```python
from build123d import *

# Parameters (mm, degrees)
MEMBER_1_DEPTH               = 1500
HOLE_WIZARD_M10_1_AT_2_COUNT = 2
HOLE_WIZARD_M10_1_AT_2_PITCH = 80
HOLE_WIZARD_M8_2_D           = 6.8
HOLE_WIZARD_M8_2_DEPTH       = 22.25
HOLE_WIZARD_M8_2_TIP         = 2.042926105


with BuildPart() as part:
    # Sketch11 → Member 1 (new body)
    with BuildSketch(Plane.YZ):
        with BuildLine():
            Line((-34, -40), (34, -40))
            ThreePointArc((34, -40), (38.242640687, -38.242640687), (40, -34))
            Line((40, -34), (40, 34))
            ThreePointArc((40, 34), (38.242640687, 38.242640687), (34, 40))
            Line((34, 40), (-34, 40))
            ThreePointArc((-34, 40), (-38.242640687, 38.242640687), (-40, 34))
            Line((-40, 34), (-40, -34))
            ThreePointArc((-40, -34), (-38.242640687, -38.242640687), (-34, -40))
        make_face()
        with BuildLine():
            Line((-34, -36), (34, -36))
            ThreePointArc((34, -36), (35.414213562, -35.414213562), (36, -34))
            Line((36, -34), (36, 34))
            ThreePointArc((36, 34), (35.414213562, 35.414213562), (34, 36))
            Line((34, 36), (-34, 36))
            ThreePointArc((-34, 36), (-35.414213562, 35.414213562), (-36, 34))
            Line((-36, 34), (-36, -34))
            ThreePointArc((-36, -34), (-35.414213562, -35.414213562), (-34, -36))
        make_face(mode=Mode.SUBTRACT)
    extrude(amount=MEMBER_1_DEPTH)

    # 草图4 → M10 间隙孔1 (revolve, cut)
    with BuildSketch(Plane(origin=(1380, 0, -36), x_dir=(0, -1, 0), z_dir=(1, 0, 0))):
        Polygon((0, 0), (0, 33.605163714), (6, 30), (6, 0), align=None)
    hole_wizard_m10_1 = revolve(axis=Axis((1380, 0, -29.65), (0, 0, -1)), mode=Mode.SUBTRACT)

    # M10 间隙孔1 at 2: M10 间隙孔1 ×2
    with Locations(*[(i * HOLE_WIZARD_M10_1_AT_2_PITCH, 0, 0) for i in range(1, HOLE_WIZARD_M10_1_AT_2_COUNT)]):
        add(hole_wizard_m10_1, mode=Mode.SUBTRACT)

    # 镜向1: M10 间隙孔1 across plane
    add(hole_wizard_m10_1.mirror(Plane.ZY.offset(-750)), mode=Mode.SUBTRACT)

    # 镜向1 copy 1 sketch → 镜向1 copy 1 (revolve, cut)
    with BuildSketch(Plane(origin=(40, 0, -36), x_dir=(0, -1, 0), z_dir=(-1, 0, 0))):
        Polygon((0, 0), (0, -33.605163714), (6, -30), (6, 0), align=None)
    revolve(axis=Axis((40, 0, -29.65), (0, 0, 1)), mode=Mode.SUBTRACT)

    # M8 螺纹孔2
    with Locations(Plane(origin=(0, 40, 0), x_dir=(-1, 0, 0), z_dir=(0, 1, 0))):
        with Locations((-100.000000009, 20), (-740.000000009, 20), (-1380.000000009, 20), (-1580.000000007, 20), (-2220.000000007, 20), (-2860.000000007, 20)):
            Hole(HOLE_WIZARD_M8_2_D / 2, depth=HOLE_WIZARD_M8_2_DEPTH)
            with Locations((0, 0, -(HOLE_WIZARD_M8_2_DEPTH + HOLE_WIZARD_M8_2_TIP / 2))):  # 118° drill point
                Cone(0, HOLE_WIZARD_M8_2_D / 2, HOLE_WIZARD_M8_2_TIP, mode=Mode.SUBTRACT)


solid = part.part
```
Geometry: final body of the model. Coordinates: model frame, mm. A direction names the side the tool comes from. Round coordinates to 2 decimals unless told otherwise and drop trailing zeros. Order: outer loops, then holes, each group sorted by start corner. A loop starts at its lowest first (then second) coordinate and runs counter-clockwise, first axis right, second up. Notation, with made-up numbers: (-17, -28.75) -> (12, -28.75) arc R15 cw to (12, -6.75) -> close; hole circle Ø9 at (24, -24). An arc over 180 degrees is marked (long way). Use CSV: the item, a comma, the result in double quotes. Start each with the question number.
1) Material intervals for line 1 along X through (y, z) = (0, -37.35); line 2 along Y through (x, z) = (414, -8.5), sorted ascending. Write a range as from..to.
2) Section B-B (x = 1339.5). Return the cut outline in (y, z), and give its area (3 significant figures).
3) Draft query along Z for faces 1 (the face through (740, 40, 0)), 2 (the face through (740, 0, -40)), 3 (the face through (740, 0, 36)). Return one class per face: +Z half, -Z half, draft (parallel to the pull), parting line (faces both ways), or undercut.
4) Set-up query: faces 4 (the face through (740, 36, 0)), 5 (the face through (740, -40, 0)). Return all of +Z, -Z, +X, -X, +Y, -Y with unobstructed straight access to the full face (end or side cutting, diameter ignored); none if empty.
5) Section A-A (z = -4). Return the cut outline in (x, y), and give its area (3 significant figures).
6) First-contact query: pin 1 Ø5.5 at (x, z) = (740, 20) entering from +Y; pin 2 Ø7 at (x, y) = (120, 0) entering from -Z. Flat tips, straight axial feed; report the tip coordinate or a pass-through.
Returned:
1,line 1,"x = 0..34, 46..114, 126..1374, 1386..1454, 1466..1500"
1,line 2,"y = -40..-36, 36..40"
2,outline,"(-40, -34) arc R6 ccw to (-34, -40) -> (34, -40) arc R6 ccw to (40, -34) -> (40, 34) arc R6 ccw to (34, 40) -> (-34, 40) arc R6 ccw to (-40, 34) -> close; hole (-36, -34) arc R2 ccw to (-34, -36) -> (34, -36) arc R2 ccw to (36, -34) -> (36, 34) arc R2 ccw to (34, 36) -> (-34, 36) arc R2 ccw to (-36, 34) -> close"
2,area,"1,190 mm²"
3,face 1,"draft"
3,face 2,"-Z half"
3,face 3,"undercut"
4,face 4,"+X, -X"
4,face 5,"+Z, -Z, +X, -X, -Y"
5,outline,"(0, -40) -> (1500, -40) -> (1500, -36) -> (0, -36) -> close; (0, 36) -> (1500, 36) -> (1500, 40) -> (0, 40) -> close"
5,area,"12,000 mm²"
6,pin 1,"stops at y = -36"
6,pin 2,"stops at z = 36"
